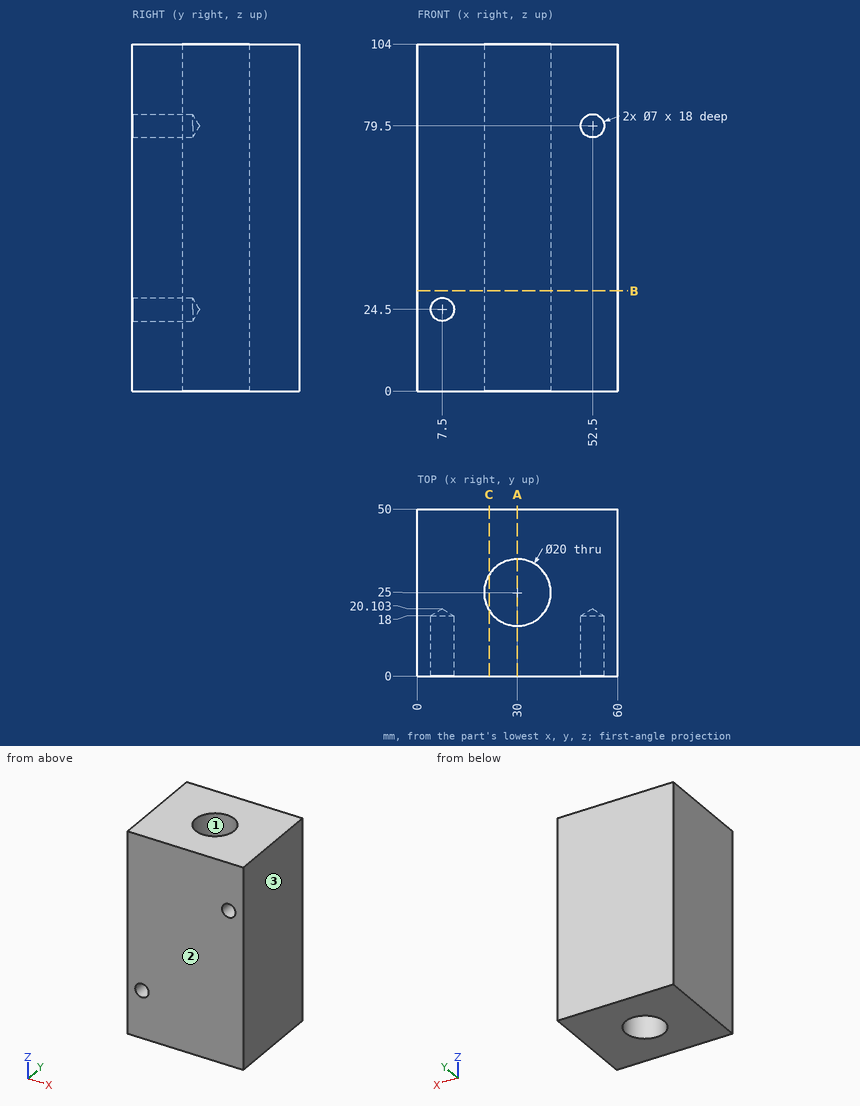
Input: dimensioned drawing with shaded views. Units: mm. Origin: part minimum x, y, z. Coordinates: 2 decimals unless noted, no trailing zeros. Order: outer loops, then holes, each group sorted by start corner. A loop starts at its lowest first (then second) coordinate and runs counter-clockwise, first axis right, second up. Notation, with made-up numbers: M 36.25,82.5 L 72.25,82.5 A26 ccw 72.25,107.5 Z; hole C 25,-24 d5. An arc over 180 degrees is marked long. Answer as CSV lines item,"result".
Q1. Draft query along X for the marked faces 1, 2 and 3. Return one class per face: pulls with the +X half, pulls with the -X half, needs draft (parallel to the pull), parting line crosses it, or undercut.
Answers:
face 1,"undercut"
face 2,"needs draft"
face 3,"pulls with the +X half"
Q2. Section C-C on x = 21.5. Return the cut outline in (y, z), and give its area (3 significant figures).
Answers:
outline,"M 0,0 L 19.73,0 L 19.73,104 L 0,104 Z; M 30.27,0 L 50,0 L 50,104 L 30.27,104 Z"
area,"4,100 mm^2"
Q3. Line query: probe 1 along Y at (x, z) = (30, 72); probe 2 along X at (y, z) = (4.75, 24.5); probe 3 along Z at (x, y) = (52.5, 10.5). Output: solid intervals per line, ascending. Write a range as [from, to].
Answers:
probe 1,"y = [0, 15], [35, 50]"
probe 2,"x = [0, 4], [11, 60]"
probe 3,"z = [0, 76], [83, 104]"
Q4. Section A-A on x = 30. Return the cut outline in (y, z), and give its area (3 significant figures).
Answers:
outline,"M 0,0 L 15,0 L 15,104 L 0,104 Z; M 35,0 L 50,0 L 50,104 L 35,104 Z"
area,"3,120 mm^2"
Q5. First-contact query: P1, Ø4, axis at x = 52.5, z = 79.5, coming from the -Y side; P2, Ø5.5, axis at x = 7.5, z = 24.5, coming from the -Y side. Flat tips, straight axial feed; report the tip coordinate or a pass-through.
Answers:
P1,"stops at y = 18.9"
P2,"stops at y = 18.45"
Q6. Section B-B on z = 30. Return the cut outline in (x, y).
Answers:
outline,"M 0,0 L 60,0 L 60,50 L 0,50 Z; hole C 30,25 d20"
